```python
from build123d import *

# Parameters (mm, degrees)
SKETCH1_R                = 12.7
BOSS_EXTRUDE1_DEPTH      = 136.525
SKETCH2_R                = 3.175
BOSS_EXTRUDE2_DEPTH      = 12.7
FILLET2_R                = 1.5875
BOSS_EXTRUDE3_DEPTH      = 63.5
BOSS_EXTRUDE3_DEPTH_BACK = 63.5
SKETCH3_R                = 12.7
FILLET3_R                = 6.35


with BuildPart() as part:
    # Sketch1 → Boss-Extrude1 (new body)
    with BuildSketch(Plane(origin=(0, 0, 0), x_dir=(0, 0, -1), z_dir=(1, 0, 0))):
        Circle(SKETCH1_R)
    extrude(amount=BOSS_EXTRUDE1_DEPTH)

    # Sketch2 → Boss-Extrude2 (add)
    with BuildSketch(Plane(origin=(136.525, 0, 0), x_dir=(0, 0, -1), z_dir=(1, 0, 0))):
        Circle(SKETCH2_R)
    extrude(amount=BOSS_EXTRUDE2_DEPTH)

    # Fillet2
    fillet2_edges = [part.edges().sort_by_distance(p)[0] for p in [
        (149.225, 0, 3.175),
    ]]
    fillet(fillet2_edges, radius=FILLET2_R)

    # Sketch3 → Boss-Extrude3 (add, two sides: drawn at the far end of the back side and taken through both)
    with BuildSketch(Plane(origin=(0, 0, 0), x_dir=(1, 0, 0), z_dir=(0, 1, 0)).offset(-BOSS_EXTRUDE3_DEPTH_BACK)):
        with Locations(Location((0, 0, 0), (0, 0, 270))):
            Circle(SKETCH3_R)
    extrude(amount=BOSS_EXTRUDE3_DEPTH + BOSS_EXTRUDE3_DEPTH_BACK)

    # Fillet3
    # the kernel refuses this fillet: 6.35 mm, written as the material it takes off along each edge
    with BuildSketch(Plane(origin=(0, -63.5, 0), x_dir=(0, 0, 1), z_dir=(-1, 0, 0))) as fillet3_piece_1:
        with BuildLine():
            CenterArc((12.7 - FILLET3_R, FILLET3_R), FILLET3_R, 270, 90)
            Line((12.7 - FILLET3_R, 0), (12.7, 0))
            Line((12.7, 0), (12.7, FILLET3_R))
        make_face()
    revolve(axis=Axis((0, -63.5, 0), (0, 1, 0)), mode=Mode.SUBTRACT)
    with BuildSketch(Plane(origin=(0, 63.5, 0), x_dir=(0, 0, 1), z_dir=(-1, 0, 0))) as fillet3_piece_2:
        with BuildLine():
            CenterArc((12.7 - FILLET3_R, -FILLET3_R), FILLET3_R, 0, 90)
            Line((12.7 - FILLET3_R, 0), (12.7, 0))
            Line((12.7, 0), (12.7, -FILLET3_R))
        make_face()
    revolve(axis=Axis((0, 63.5, 0), (0, 1, 0)), mode=Mode.SUBTRACT)


solid = part.part
```
For this review, take the finished solid that the model builds, in its own axes (mm). A direction names the side the tool comes from. Round coordinates to 2 decimals unless told otherwise and drop trailing zeros. Write each loop counter-clockwise with the first axis right and the second up, starting at its lowest first coordinate (ties: lowest second). Pieces come first, ordered by that corner, then holes. Notation, with made-up numbers: (-8.75, 70) - (-0.75, 70) arc R6 cw to (-0.75, 79) - close; hole circle Ø3 at (-25.5, 16). An arc over 180 degrees is marked (long way). Put each result on its own line as item: value.
Q1. We need section A-A (y = 26). Give the boundary of the cut face in (x, z), and give its area (3 significant figures).
Solved:
outline: circle Ø25.4 at (0, 0)
area: 507 mm2
Q2. We need section C-C (y = -10). Give the boundary of the cut face in (x, z) (3 decimals), and give its area (3 significant figures).
Solved:
outline: (10, -7.829) - (136.525, -7.829) - (136.525, 7.829) - (10, 7.829) arc R12.7 ccw (long way) to start
area: 2,460 mm2
Q3. Wall thickness on probe 1 along X at (y, z) = (-51, 1); probe 2 along Z at (x, y) = (118.5, 0.5); probe 3 along Y at (x, z) = (125.5, 10.75): over which ranges is each line inside the solid? List them lowest first.
Solved:
probe 1: x = -12.66 to 12.66
probe 2: z = -12.69 to 12.69
probe 3: y = -6.76 to 6.76
Q4. Insertion check: pin 1 Ø1 at (y, z) = (7.5, -8.5) entering from +X (3 decimals); pin 2 Ø1 at (y, z) = (-33.5, 1) entering from +X; pin 3 Ø1.5 at (y, z) = (-49, 8) entering from +X. Each pin has a flat end and moves straight along its axis. Give the tip position at first contact, or say it passes through.
Solved:
pin 1: stops at x = 136.525
pin 2: stops at x = 12.69
pin 3: stops at x = 10.43
Q5. Machinability: for faces 1 (the face through (0, 63.5, 0)), 2 (the face through (-12.4, -0.8, -2.75)), 3 (the face through (142, -3.1, 0.69)), which of the approach directions +Z, -Z, +X, -X, +Y, -Y give a long, thin tool a straight path to every point of the face, cutting with its end or side? Answer none if there is none.
Solved:
face 1: +Z, -Z, +X, -X, +Y
face 2: none
face 3: +X
